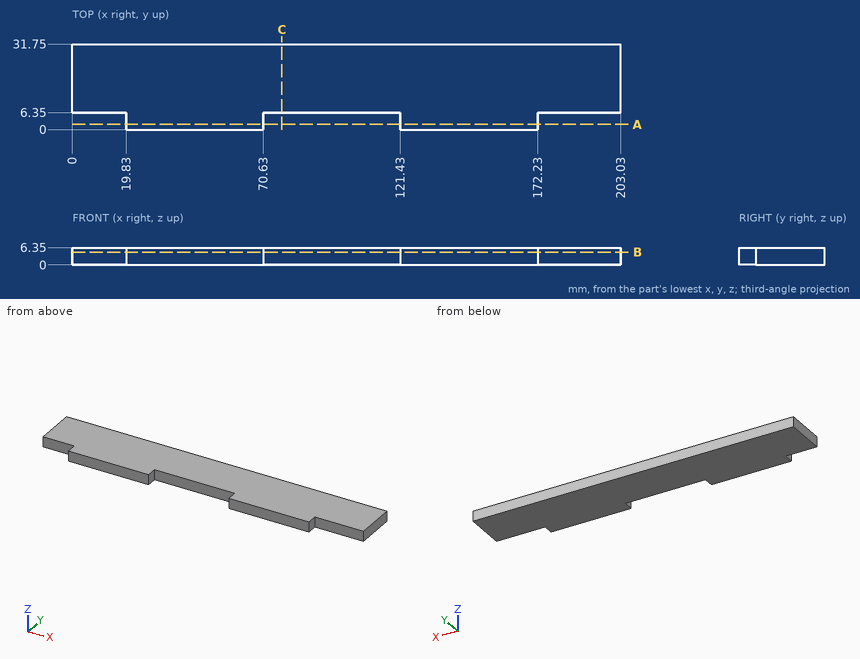
Check sheet for the drawn part. Datum: minimum x, y, z corner. Units: mm. Round coordinates to 2 decimals unless told otherwise and drop trailing zeros. Write each loop counter-clockwise with the first axis right and the second up, starting at its lowest first coordinate (ties: lowest second). Pieces come first, ordered by that corner, then holes. Notation, with made-up numbers: (32, 89.5) -> (50, 89.5) arc R23 cw to (50, 98.5) -> close; hole circle Ø9 at (77, 20.5). An arc over 180 degrees is marked (long way). One line per item, written item: value. Start each with the question number.
(1) Cross-section at A-A, the plane y = 2. Record the cut outline in (x, z), and give its area (3 significant figures).
(2) Scan lines: line 1 (X direction, y = 4, z = 4.25); line 2 (Y direction, x = 176, z = 4.5). Record each from-to range of solid material in increasing order. Write a range as [from, to].
(3) Cross-section at C-C, the plane x = 77.5. Record the cut outline in (y, z), and give its area (3 significant figures).
(4) Cross-section at B-B, the plane z = 4.75. Record the cut outline in (x, y), and give its area (3 significant figures).
(5) Go/stop test with flat-tipped pins: pin 1 Ø3 at (y, z) = (4.5, 5) entering from -X; pin 2 Ø12 at (x, y) = (80, 3.5) entering from -Z; pin 3 Ø3 at (x, z) = (84.5, 5) entering from -Y. Record where each tip stops, or that it passes through.
Answer:
1. outline: (19.83, 0) -> (70.63, 0) -> (70.63, 6.35) -> (19.83, 6.35) -> close; (121.43, 0) -> (172.23, 0) -> (172.23, 6.35) -> (121.43, 6.35) -> close
1. area: 645 mm²
2. line 1: [19.83, 70.63], [121.43, 172.23]
2. line 2: [6.35, 31.75]
3. outline: (6.35, 0) -> (31.75, 0) -> (31.75, 6.35) -> (6.35, 6.35) -> close
3. area: 161 mm²
4. outline: (0, 6.35) -> (19.83, 6.35) -> (19.83, 0) -> (70.63, 0) -> (70.63, 6.35) -> (121.43, 6.35) -> (121.43, 0) -> (172.23, 0) -> (172.23, 6.35) -> (203.03, 6.35) -> (203.03, 31.75) -> (0, 31.75) -> close
4. area: 5,800 mm²
5. pin 1: x = 19.83
5. pin 2: z = 0
5. pin 3: y = 6.35
